```python
from build123d import *

# Parameters (mm, degrees)
F0_R      = 31.75
F0_R_2    = 25.4
F1_DEPTH  = 25.4
F2_R      = 86.36
F3_DEPTH  = 25.4
F3_FACE_R = 25.4
F4_DEPTH  = 50.8
F5_R      = 86.36
F5_R_2    = 25.4
F6_DEPTH  = 25.4


with BuildPart() as f1:
    # F0 (on Front) → F1 (new body)
    with BuildSketch(Plane.XZ):
        with BuildLine():
            ThreePointArc((-6.35, 43.99409), (0, 44.45), (6.35, 43.99409))
            ThreePointArc((6.35, 43.99409), (5.51657, 63.657692), (0, 82.55))
            ThreePointArc((0, 82.55), (-5.51657, 63.657692), (-6.35, 43.99409))
        make_face()
        with BuildLine():
            ThreePointArc((-27.496306, 34.925), (-22.225, 38.494829), (-16.497784, 41.275))
            ThreePointArc((-16.497784, 41.275), (-27.051357, 57.887463), (-41.275, 71.490397))
            ThreePointArc((-41.275, 71.490397), (-36.606335, 52.370894), (-27.496306, 34.925))
        make_face()
        with BuildLine():
            ThreePointArc((-41.275, 16.497784), (-38.494829, 22.225), (-34.925, 27.496307))
            ThreePointArc((-34.925, 27.496307), (-52.370894, 36.606335), (-71.490397, 41.275))
            ThreePointArc((-71.490397, 41.275), (-57.887463, 27.051357), (-41.275, 16.497784))
        make_face()
        with BuildLine():
            ThreePointArc((-43.99409, -6.35), (-44.45, 0), (-43.99409, 6.35))
            ThreePointArc((-43.99409, 6.35), (-63.657692, 5.51657), (-82.55, 0))
            ThreePointArc((-82.55, 0), (-63.657692, -5.51657), (-43.99409, -6.35))
        make_face()
        with BuildLine():
            ThreePointArc((-71.490397, -41.275), (-52.370894, -36.606335), (-34.925, -27.496306))
            ThreePointArc((-34.925, -27.496306), (-38.494829, -22.225), (-41.275, -16.497784))
            ThreePointArc((-41.275, -16.497784), (-57.887463, -27.051357), (-71.490397, -41.275))
        make_face()
        with BuildLine():
            ThreePointArc((-41.275, -71.490397), (-27.051357, -57.887463), (-16.497784, -41.275))
            ThreePointArc((-16.497784, -41.275), (-22.225, -38.494829), (-27.496307, -34.925))
            ThreePointArc((-27.496307, -34.925), (-36.606335, -52.370894), (-41.275, -71.490397))
        make_face()
        with BuildLine():
            ThreePointArc((0, -82.55), (5.51657, -63.657692), (6.35, -43.99409))
            ThreePointArc((6.35, -43.99409), (0, -44.45), (-6.35, -43.99409))
            ThreePointArc((-6.35, -43.99409), (-5.51657, -63.657692), (0, -82.55))
        make_face()
        with BuildLine():
            ThreePointArc((41.275, -71.490397), (36.606335, -52.370894), (27.496306, -34.925))
            ThreePointArc((27.496306, -34.925), (22.225, -38.494829), (16.497784, -41.275))
            ThreePointArc((16.497784, -41.275), (27.051357, -57.887463), (41.275, -71.490397))
        make_face()
        with BuildLine():
            ThreePointArc((71.490397, -41.275), (57.887463, -27.051357), (41.275, -16.497784))
            ThreePointArc((41.275, -16.497784), (38.494829, -22.225), (34.925, -27.496307))
            ThreePointArc((34.925, -27.496307), (52.370894, -36.606335), (71.490397, -41.275))
        make_face()
        with BuildLine():
            ThreePointArc((43.99409, 6.35), (44.335876, 3.183173), (44.45, 0))
            ThreePointArc((44.45, 0), (44.335876, -3.183173), (43.99409, -6.35))
            ThreePointArc((43.99409, -6.35), (63.657692, -5.51657), (82.55, 0))
            ThreePointArc((82.55, 0), (63.657692, 5.51657), (43.99409, 6.35))
        make_face()
        with BuildLine():
            ThreePointArc((34.925, 27.496306), (38.494829, 22.225), (41.275, 16.497784))
            ThreePointArc((41.275, 16.497784), (57.887463, 27.051357), (71.490397, 41.275))
            ThreePointArc((71.490397, 41.275), (52.370894, 36.606335), (34.925, 27.496306))
        make_face()
        with BuildLine():
            ThreePointArc((16.497784, 41.275), (22.225, 38.494829), (27.496307, 34.925))
            ThreePointArc((27.496307, 34.925), (36.606335, 52.370894), (41.275, 71.490397))
            ThreePointArc((41.275, 71.490397), (27.051357, 57.887463), (16.497784, 41.275))
        make_face()
        with BuildLine():
            ThreePointArc((43.99409, -6.35), (44.335876, -3.183173), (44.45, 0))
            ThreePointArc((44.45, 0), (44.335876, 3.183173), (43.99409, 6.35))
            ThreePointArc((43.99409, 6.35), (42.935403, 11.504506), (41.275, 16.497784))
            ThreePointArc((41.275, 16.497784), (38.494829, 22.225), (34.925, 27.496306))
            ThreePointArc((34.925, 27.496306), (31.430896, 31.430896), (27.496307, 34.925))
            ThreePointArc((27.496307, 34.925), (22.225, 38.494829), (16.497784, 41.275))
            ThreePointArc((16.497784, 41.275), (11.504507, 42.935403), (6.35, 43.99409))
            ThreePointArc((6.35, 43.99409), (0, 44.45), (-6.35, 43.99409))
            ThreePointArc((-6.35, 43.99409), (-11.504506, 42.935403), (-16.497784, 41.275))
            ThreePointArc((-16.497784, 41.275), (-22.225, 38.494829), (-27.496306, 34.925))
            ThreePointArc((-27.496306, 34.925), (-31.430896, 31.430896), (-34.925, 27.496307))
            ThreePointArc((-34.925, 27.496307), (-38.494829, 22.225), (-41.275, 16.497784))
            ThreePointArc((-41.275, 16.497784), (-42.935403, 11.504507), (-43.99409, 6.35))
            ThreePointArc((-43.99409, 6.35), (-44.45, 0), (-43.99409, -6.35))
            ThreePointArc((-43.99409, -6.35), (-42.935403, -11.504506), (-41.275, -16.497784))
            ThreePointArc((-41.275, -16.497784), (-38.494829, -22.225), (-34.925, -27.496306))
            ThreePointArc((-34.925, -27.496306), (-31.430896, -31.430896), (-27.496307, -34.925))
            ThreePointArc((-27.496307, -34.925), (-22.225, -38.494829), (-16.497784, -41.275))
            ThreePointArc((-16.497784, -41.275), (-11.504507, -42.935403), (-6.35, -43.99409))
            ThreePointArc((-6.35, -43.99409), (0, -44.45), (6.35, -43.99409))
            ThreePointArc((6.35, -43.99409), (11.504506, -42.935403), (16.497784, -41.275))
            ThreePointArc((16.497784, -41.275), (22.225, -38.494829), (27.496306, -34.925))
            ThreePointArc((27.496306, -34.925), (31.430896, -31.430896), (34.925, -27.496307))
            ThreePointArc((34.925, -27.496307), (38.494829, -22.225), (41.275, -16.497784))
            ThreePointArc((41.275, -16.497784), (42.935403, -11.504507), (43.99409, -6.35))
        make_face()
        Circle(F0_R, mode=Mode.SUBTRACT)
        Circle(F0_R)
        Circle(F0_R_2, mode=Mode.SUBTRACT)
    extrude(amount=F1_DEPTH)

    # F2 (on Front) → F3 (join)
    with BuildSketch(Plane.XZ):
        Circle(F2_R)
    extrude(amount=-F3_DEPTH)

    # F3_face (on face) → F4 (cut)
    with BuildSketch(Plane.XZ):
        Circle(F3_FACE_R)
    extrude(amount=-F4_DEPTH, mode=Mode.SUBTRACT)

    # F5 (on face) → F6 (join)
    with BuildSketch(Plane.XZ.offset(25.4)):
        Circle(F5_R)
        Circle(F5_R_2, mode=Mode.SUBTRACT)
    extrude(amount=F6_DEPTH)


solid = f1.part
```
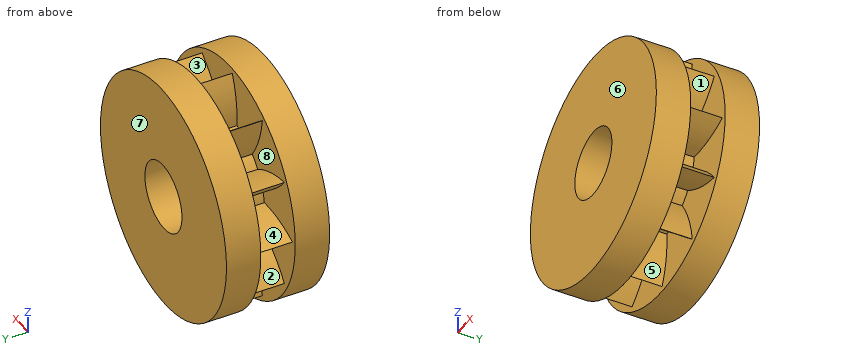
Geometry: final body of the model. Coordinates: model frame, mm. Face numbers are marked on the shaded views. A direction names the side the tool comes from. Round coordinates to 2 decimals unless told otherwise and drop trailing zeros. Loops run counter-clockwise (first coordinate to the right, second up) from the corner with the lowest first, then second, coordinate; pieces in that order, holes last.
Item 1: Line query: L1, parallel to X at y = -4.5, z = -36; L2, parallel to Z at x = -62, y = -16.5; L3, parallel to Z at x = -49.5, y = -18.5. Output: solid intervals per line, ascending.
Checked values:
L1: x = -67.19 to -50.81, -28.22 to 28.22, 50.81 to 67.19
L2: z = -39.57 to -30.66, -5.77 to 5.77, 30.66 to 39.57
L3: z = -35.46 to -21.02, -6.6 to 6.6, 21.02 to 35.46
Item 2: Section B-B, the plane x = 57.5. Output: boundary loops of the cut face in (y, z).
Checked values:
outline: (-50.8, -64.43) - (-25.4, -64.43) - (-25.4, -38.35) - (0, -38.35) - (0, -64.43) - (25.4, -64.43) - (25.4, 64.43) - (0, 64.43) - (0, 38.35) - (-25.4, 38.35) - (-25.4, 64.43) - (-50.8, 64.43) - close; hole (-25.4, -26.74) - (0, -26.74) - (0, -6.29) - (-25.4, -6.29) - close; hole (-25.4, 6.29) - (0, 6.29) - (0, 26.74) - (-25.4, 26.74) - close
Item 3: Section C-C, the plane z = 37.5. Output: boundary loops of the cut face in (x, y), plus the area to 3 significant figures.
Checked values:
outline: (-77.79, -50.8) - (77.79, -50.8) - (77.79, -25.4) - (68.49, -25.4) - (68.49, 0) - (77.79, 0) - (77.79, 25.4) - (-77.79, 25.4) - (-77.79, 0) - (-68.49, 0) - (-68.49, -25.4) - (-77.79, -25.4) - close; hole (-54.86, -25.4) - (-29.2, -25.4) - (-29.2, 0) - (-54.86, 0) - close; hole (29.2, -25.4) - (54.86, -25.4) - (54.86, 0) - (29.2, 0) - close
area: 10,100 mm2
Item 4: Mould query, pull axis Y, two halves, no side actions, for the marked faces 5, 6, 7 and 8. Classes: released by +Y, released by -Y, zero draft, split by the parting line, or undercut.
Checked values:
face 5: undercut
face 6: released by -Y
face 7: released by +Y
face 8: undercut
Item 5: Section D-D, the plane y = 5. Output: boundary loops of the cut face in (x, z).
Checked values:
outline: circle Ø172.72 at (0, 0); hole circle Ø50.8 at (0, 0)
Item 6: Section A-A, the plane z = 4. Output: boundary loops of the cut face in (x, y), plus the area to 3 significant figures.
Checked values:
outline: (-86.27, -50.8) - (-25.08, -50.8) - (-25.08, 25.4) - (-86.27, 25.4) - (-86.27, 0) - (-70.84, 0) - (-70.84, -25.4) - (-86.27, -25.4) - close; (25.08, -50.8) - (86.27, -50.8) - (86.27, -25.4) - (70.84, -25.4) - (70.84, 0) - (86.27, 0) - (86.27, 25.4) - (25.08, 25.4) - close
area: 8,540 mm2
Item 7: Reachability of the marked faces 1, 2, 3 and 4 from +Z, -Z, +X, -X, +Y, -Y: full face, straight path, thin tool, end or side. Return the list, or none.
Checked values:
face 1: +X
face 2: -X
face 3: +Z
face 4: none
Item 8: Contact query for flat-ended pins moving along their axis: P1, Ø3, axis at x = 16.5, y = 9.5, coming from the +Z side; P2, Ø10, axis at y = 14, z = -62, coming from the -X side; P3, Ø1, axis at y = -3, z = -59, coming from the +X side. Output: stop coordinate, or through.
Checked values:
P1: stops at z = 85.05
P2: stops at x = -64.88
P3: stops at x = 38.92
